from build123d import *

# Parameters (mm, degrees)
CROQUIS1_W              = 50
CROQUIS1_H              = 97
SALIENTE_EXTRUIR1_DEPTH = 5
CROQUIS2_R              = 3.6
CROQUIS2_R_2            = 2.55
CORTAR_EXTRUIR2_DEPTH   = 6
CROQUIS4_R              = 6
CROQUIS4_R_2            = 5.05
CORTAR_EXTRUIR3_DEPTH   = 2
CROQUIS5_R              = 1.55
CROQUIS5_W              = 6
CROQUIS5_H              = 4.2
CORTAR_EXTRUIR4_DEPTH   = 6
CORTAR_EXTRUIR6_DEPTH   = 6
CROQUIS14_R             = 3
CORTAR_EXTRUIR9_DEPTH   = 2.5
CROQUIS18_R             = 10.5
CROQUIS18_R_2           = 1.525
CORTAR_EXTRUIR10_DEPTH  = 6
CROQUIS20_W             = 42
CROQUIS20_H             = 25.956058456
CORTAR_EXTRUIR11_DEPTH  = 6


with BuildPart() as part:
    # Croquis1 → Saliente-Extruir1 (new body)
    with BuildSketch(Plane(origin=(0, 0, 0), x_dir=(1, 0, 0), z_dir=(0, 1, 0))):
        Rectangle(CROQUIS1_W, CROQUIS1_H)
    extrude(amount=SALIENTE_EXTRUIR1_DEPTH)

    # Croquis2 → Cortar-Extruir2 (cut, through all)
    with BuildSketch(Plane(origin=(0, 5, 0), x_dir=(1, 0, 0), z_dir=(0, 1, 0))):
        with Locations((-15, 32.45)):
            Circle(CROQUIS2_R)
        with Locations((15, 32.45)):
            Circle(CROQUIS2_R)
        with Locations((15, -19.45)):
            Circle(CROQUIS2_R_2)
        with Locations((-15, -19.45)):
            Circle(CROQUIS2_R_2)
    extrude(amount=-CORTAR_EXTRUIR2_DEPTH, mode=Mode.SUBTRACT)

    # Croquis4 → Cortar-Extruir3 (cut)
    with BuildSketch(Plane.XZ):
        with Locations((15, -32.45)):
            Circle(CROQUIS4_R)
        with Locations((-15, -32.45)):
            Circle(CROQUIS4_R)
        with Locations((-15, 19.45)):
            Circle(CROQUIS4_R_2)
        with Locations((15, 19.45)):
            Circle(CROQUIS4_R_2)
    extrude(amount=-CORTAR_EXTRUIR3_DEPTH, mode=Mode.SUBTRACT)

    # Croquis5 → Cortar-Extruir4 (cut, through all)
    with BuildSketch(Plane(origin=(0, 5, 0), x_dir=(1, 0, 0), z_dir=(0, 1, 0))):
        with Locations((0, 43.5)):
            Circle(CROQUIS5_R)
        with Locations((-11, 43.5)):
            Rectangle(CROQUIS5_W, CROQUIS5_H)
        with Locations((11, 43.5)):
            Rectangle(CROQUIS5_W, CROQUIS5_H)
    cortar_extruir4 = extrude(amount=-CORTAR_EXTRUIR4_DEPTH, mode=Mode.SUBTRACT)

    # Croquis8 → Cortar-Extruir6 (cut, through all)
    with BuildSketch(Plane(origin=(0, 5, 0), x_dir=(1, 0, 0), z_dir=(0, 1, 0))):
        with BuildLine():
            Line((-11.878679656, 45.6), (-10.121320344, 45.6))
            ThreePointArc((-10.121320344, 45.6), (-8.010608171, 45.610503119), (-7.979099854, 43.5))
            ThreePointArc((-7.979099854, 43.5), (-8.010608171, 41.389496881), (-10.121320344, 41.4))
            Line((-10.121320344, 41.4), (-11.878679656, 41.4))
            ThreePointArc((-11.878679656, 41.4), (-13.989391829, 41.389496881), (-14.020900146, 43.5))
            ThreePointArc((-14.020900146, 43.5), (-13.989391829, 45.610503119), (-11.878679656, 45.6))
        make_face()
        with BuildLine():
            Line((10.121320344, 41.4), (11.878679656, 41.4))
            ThreePointArc((11.878679656, 41.4), (13.989391829, 41.389496881), (14.020900146, 43.5))
            ThreePointArc((14.020900146, 43.5), (13.989391829, 45.610503119), (11.878679656, 45.6))
            Line((11.878679656, 45.6), (10.121320344, 45.6))
            ThreePointArc((10.121320344, 45.6), (8.010608171, 45.610503119), (7.979099854, 43.5))
            ThreePointArc((7.979099854, 43.5), (8.010608171, 41.389496881), (10.121320344, 41.4))
        make_face()
    cortar_extruir6 = extrude(amount=-CORTAR_EXTRUIR6_DEPTH, mode=Mode.SUBTRACT)

    # Simetría1: Cortar-Extruir4, Cortar-Extruir6 across plane
    add(cortar_extruir4.mirror(Plane.XY.offset(-26)), mode=Mode.SUBTRACT)
    add(cortar_extruir6.mirror(Plane.XY.offset(-26)), mode=Mode.SUBTRACT)

    # Croquis14 → Cortar-Extruir9 (cut)
    with BuildSketch(Plane(origin=(0, 5, 0), x_dir=(1, 0, 0), z_dir=(0, 1, 0))):
        with Locations((0, 8.5)):
            Circle(CROQUIS14_R)
    extrude(amount=-CORTAR_EXTRUIR9_DEPTH, mode=Mode.SUBTRACT)

    # Croquis18 → Cortar-Extruir10 (cut, through all)
    with BuildSketch(Plane(origin=(0, 5, 0), x_dir=(1, 0, 0), z_dir=(0, 1, 0))):
        with Locations((0, -35.5)):
            Circle(CROQUIS18_R)
        with Locations((9.75, -45.5)):
            Circle(CROQUIS18_R_2)
        with Locations((-9.75, -45.5)):
            Circle(CROQUIS18_R_2)
        with Locations((9.75, -25.5)):
            Circle(CROQUIS18_R_2)
        with Locations((-9.75, -25.5)):
            Circle(CROQUIS18_R_2)
    extrude(amount=-CORTAR_EXTRUIR10_DEPTH, mode=Mode.SUBTRACT)

    # Croquis20 → Cortar-Extruir11 (cut, through all)
    with BuildSketch(Plane.XZ):
        with Locations((0, 37.343359165)):
            Rectangle(CROQUIS20_W, CROQUIS20_H)
    extrude(amount=-CORTAR_EXTRUIR11_DEPTH, mode=Mode.SUBTRACT)


solid = part.part
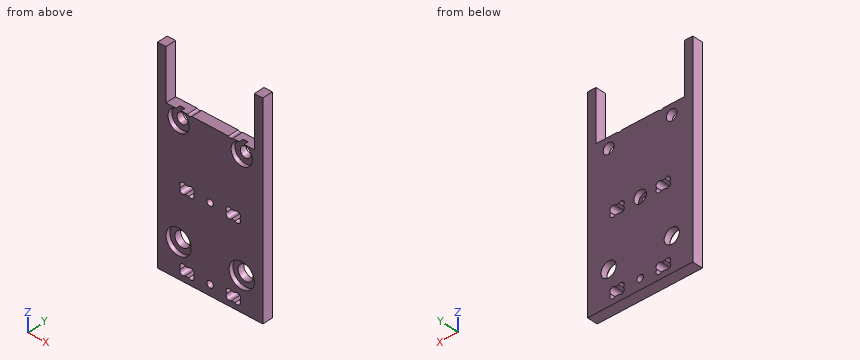
Read the model definition and answer for the solid it produces. Units are mm, in the model's axes. Coordinates: 2 decimals unless noted, no trailing zeros. Order: outer loops, then holes, each group sorted by start corner. A loop starts at its lowest first (then second) coordinate and runs counter-clockwise, first axis right, second up. Notation, with made-up numbers: (74.25, -18) - (103.25, -18) arc R20 ccw to (103.25, 5) - close; hole circle Ø9 at (68.25, 6). An arc over 180 degrees is marked (long way). Use one line per item in the form item = value.
(1) Given pin 1 Ø1.5 at (x, y) = (-18, 1.5) entering from +Z; pin 2 Ø3 at (x, z) = (-13.5, 18) entering from -Y; pin 3 Ø7 at (x, z) = (15, -32.45) entering from +Y; pin 4 Ø3.5 at (x, z) = (0, -8.5) entering from +Y, each flat-ended and moving along its own axis, determine where each tip first touches the part or whether it passes through.
Computed values:
pin_1 = 24.37
pin_2 = 2
pin_3 = through
pin_4 = 2.5
(2) Section B-B, the plane z = -32.45 is taken. Give the vertices of the cut face in (x, y).
Computed values:
outline = (-25, 0) - (-21, 0) - (-21, 2) - (-18.6, 2) - (-18.6, 5) - (-25, 5) - close; (-11.4, 2) - (-9, 2) - (-9, 0) - (9, 0) - (9, 2) - (11.4, 2) - (11.4, 5) - (-11.4, 5) - close; (18.6, 2) - (21, 2) - (21, 0) - (25, 0) - (25, 5) - (18.6, 5) - close
(3) Straight lines are drawn through the part: L1, parallel to Z at x = -15, y = 3.8; L2, parallel to X at y = 0.5, z = 19.45; L3, parallel to Z at x = 0, y = 1.25. For each, find the intervals that lie inside material, in ascending order.
Computed values:
L1 = -48.5 to -36.05, -28.85 to 16.9, 22 to 24.37
L2 = -25 to -20.05, -9.95 to 9.95, 20.05 to 25
L3 = -48.5 to -45.05, -41.95 to -10.05, -6.95 to 24.37
(4) Section D-D, the plane y = 3.8 is taken. Give the number of separate pieces and of enclosed holes in the cut face, then the cut area to 3 significant figures.
Computed values:
separate_pieces = 1
enclosed_holes = 10
area = 3,560 mm²
(5) Section C-C, the plane z = 19.45 is taken. Give the vertices of the cut face in (x, y).
Computed values:
outline = (-25, 0) - (-20.05, 0) - (-20.05, 2) - (-17.55, 2) - (-17.55, 5) - (-25, 5) - close; (-12.45, 2) - (-9.95, 2) - (-9.95, 0) - (9.95, 0) - (9.95, 2) - (12.45, 2) - (12.45, 5) - (-12.45, 5) - close; (17.55, 2) - (20.05, 2) - (20.05, 0) - (25, 0) - (25, 5) - (17.55, 5) - close
(6) Section A-A, the plane x = 0 is taken. Give the vertices of the cut face in (y, z), then the cut area to 3 significant figures.
Computed values:
outline = (0, -48.5) - (5, -48.5) - (5, -45.05) - (0, -45.05) - close; (0, -41.95) - (5, -41.95) - (5, -11.5) - (2.5, -11.5) - (2.5, -10.05) - (0, -10.05) - close; (0, -6.95) - (2.5, -6.95) - (2.5, -5.5) - (5, -5.5) - (5, 24.37) - (0, 24.37) - close
area = 326 mm²
